Could you check a few things on this model? Use its own coordinates, in mm. Face numbers are marked on the shaded views. A direction names the side the tool comes from. Give positions to 0.01 mm unless a question says otherwise; leave off trailing zeros. Order: outer loops, then holes, each group sorted by start corner. A loop starts at its lowest first (then second) coordinate and runs counter-clockwise, first axis right, second up. Notation, with made-up numbers: (83, 13.25) -> (89, 13.25) arc R15 ccw to (89, 21.25) -> close; hole circle Ø11 at (19.25, -29.75). An arc over 180 degrees is marked (long way). Write each question's results on one line, items separated by ' | '.
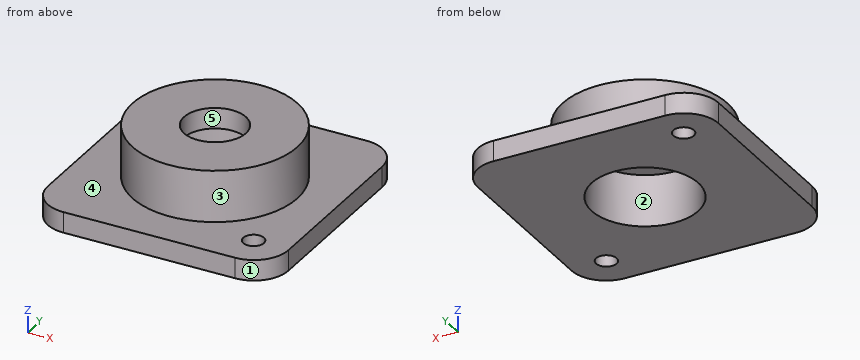
```python
from build123d import *

# Parameters (mm, degrees)
SKETCH_W      = 35
SKETCH_H      = 35
SKETCH_R      = 7.75
SKETCH_R_2    = 1.5
PAD_DEPTH     = 3
SKETCH001_R   = 12
SKETCH001_R_2 = 7.75
PAD001_DEPTH  = 4.5
SKETCH002_R   = 12
SKETCH002_R_2 = 4.5
PAD002_DEPTH  = 3
FILLET_R      = 5


with BuildPart() as part:
    # Sketch → Pad (new body)
    with BuildSketch(Plane.XY):
        Rectangle(SKETCH_W, SKETCH_H)
        Circle(SKETCH_R, mode=Mode.SUBTRACT)
        with Locations((-12.375262, 12.375262)):
            Circle(SKETCH_R_2, mode=Mode.SUBTRACT)
        with Locations((12.373476, -12.373476)):
            Circle(SKETCH_R_2, mode=Mode.SUBTRACT)
    extrude(amount=PAD_DEPTH)

    # Sketch001 (on Face9 of Pad) → Pad001 (join)
    with BuildSketch(Plane.XY.offset(3)):
        Circle(SKETCH001_R)
        Circle(SKETCH001_R_2, mode=Mode.SUBTRACT)
    extrude(amount=PAD001_DEPTH)

    # Sketch002 (on Face10 of Pad001) → Pad002 (join)
    with BuildSketch(Plane.XY.offset(7.5)):
        Circle(SKETCH002_R)
        Circle(SKETCH002_R_2, mode=Mode.SUBTRACT)
    extrude(amount=PAD002_DEPTH)

    # Fillet
    fillet_edges = [part.edges().sort_by_distance(p)[0] for p in [
        (17.5, -17.5, 1.5),
        (17.5, 17.5, 1.5),
        (-17.5, -17.5, 1.5),
        (-17.5, 17.5, 1.5),
    ]]
    fillet(fillet_edges, radius=FILLET_R)


solid = part.part
```
Q1. I need wall thicknesses on line 1 along Y through (x, z) = (0, 4.5); line 2 along Y through (x, z) = (0, 8.8); line 3 along X through (y, z) = (-0.5, 5.5). Which ranges of each line are inside material? Lowest first, please.
Here are the results:
line 1: y = -12 to -7.75, 7.75 to 12 | line 2: y = -12 to -4.5, 4.5 to 12 | line 3: x = -11.99 to -7.73, 7.73 to 11.99
Q2. Thinking about a two-plate mould opening in Y: for the marked faces 3, 4 and 5, which applies, +Y half, -Y half, draft (parallel to the pull), parting line (faces both ways), or undercut?
Here are the results:
face 3: parting line | face 4: draft | face 5: undercut
Q3. Suppose I cut it at C-C on z = 1.5. Please give me the cut outline in (x, y).
Here are the results:
outline: (-17.5, -12.5) arc R5 ccw to (-12.5, -17.5) -> (12.5, -17.5) arc R5 ccw to (17.5, -12.5) -> (17.5, 12.5) arc R5 ccw to (12.5, 17.5) -> (-12.5, 17.5) arc R5 ccw to (-17.5, 12.5) -> close; hole circle Ø3 at (-12.38, 12.38); hole circle Ø15.5 at (0, 0); hole circle Ø3 at (12.37, -12.37)
Q4. Suppose I cut it at D-D on x = -7. Please give me the cut outline in (y, z), and give its area (3 significant figures).
Here are the results:
outline: (-17.5, 0) -> (-3.33, 0) -> (-3.33, 7.5) -> (3.33, 7.5) -> (3.33, 0) -> (17.5, 0) -> (17.5, 3) -> (9.75, 3) -> (9.75, 10.5) -> (-9.75, 10.5) -> (-9.75, 3) -> (-17.5, 3) -> close | area: 201 mm²
Q5. For the marked faces 1 and 2, which set-ups out of +Z, -Z, +X, -X, +Y, -Y let a thin tool reach every point of the face, with its end or its side?
Here are the results:
face 1: +Z, -Z, +X, -Y | face 2: -Z
Q6. Suppose I cut it at A-A on x = 0. Please give me the cut outline in (y, z).
Here are the results:
outline: (-17.5, 0) -> (-7.75, 0) -> (-7.75, 7.5) -> (-4.5, 7.5) -> (-4.5, 10.5) -> (-12, 10.5) -> (-12, 3) -> (-17.5, 3) -> close; (4.5, 7.5) -> (7.75, 7.5) -> (7.75, 0) -> (17.5, 0) -> (17.5, 3) -> (12, 3) -> (12, 10.5) -> (4.5, 10.5) -> close
Q7. I'm going to push flat-ended pins straight in: pin 1 Ø2 at (x, z) = (8, 7) entering from -Y; pin 2 Ø4 at (x, z) = (-1.5, 7.5) entering from +Y; pin 3 Ø6 at (y, z) = (-14, 9) entering from +X; pin 4 Ø5 at (x, y) = (-12.38, 12.38) entering from -Z. Where does each tip first touch, or does it pass through?
Here are the results:
pin 1: stops at y = -9.75 | pin 2: stops at y = 12 | pin 3: stops at x = 4.8 | pin 4: stops at z = 0
